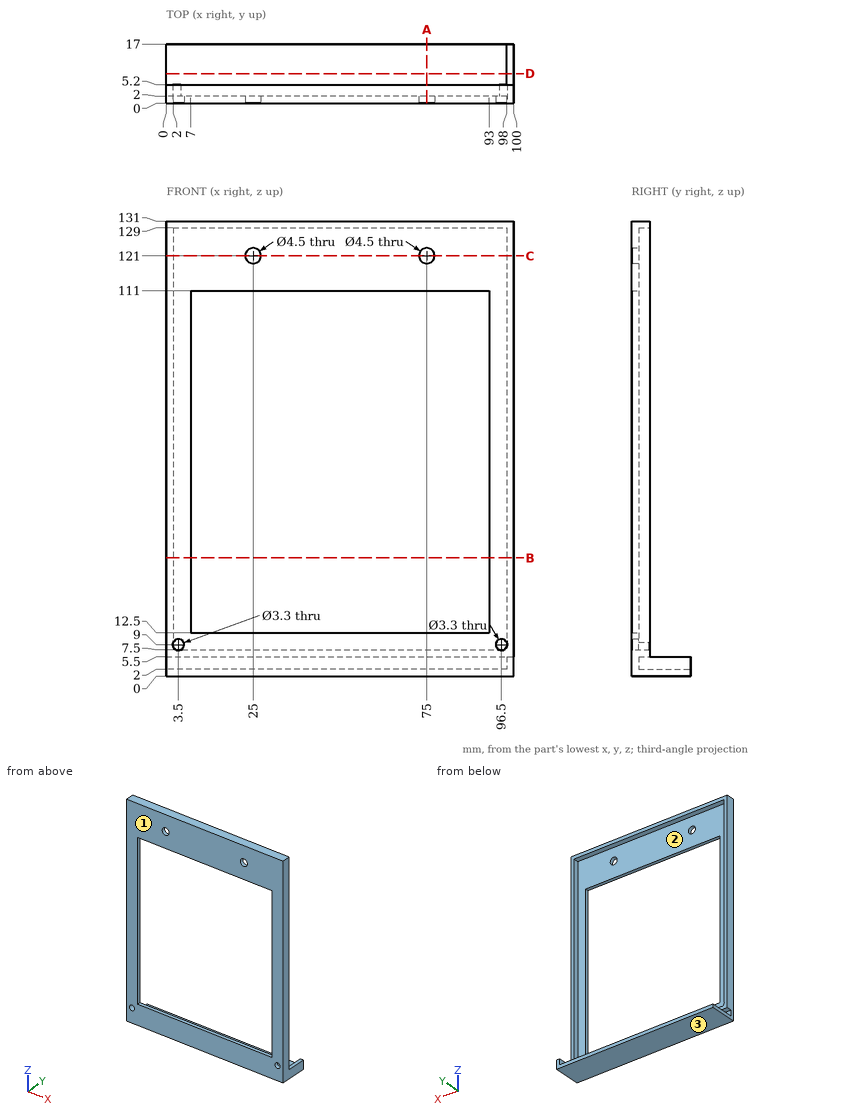
Could you check a few things on this drawing? It's one solid part, dimensions in mm from its lowest x, y, z. Give positions to 0.01 mm unless a question says otherwise; leave off trailing zeros. Write each loop counter-clockwise with the first axis right and the second up, starting at its lowest first coordinate (ties: lowest second). Pieces come first, ordered by that corner, then holes. Notation, with made-up numbers: (-12.5, 12) -> (5.5, 12) arc R19 cw to (5.5, 39) -> close; hole circle Ø7 at (-19, 57.5). An arc over 180 degrees is marked (long way). Answer as CSV lines item,"result". Start each with the question number.
(1) I'm going to push flat-ended pins straight in: pin 1 Ø4 at (x, y) = (16, 10) entering from +Z; pin 2 Ø1 at (x, z) = (34, 3.5) entering from +Y; pin 3 Ø2 at (x, y) = (99, 9) entering from +Z. Where does each tip first touch, or does it pass through?
(2) If we section it at B-B, the plane z = 34: Write out the boundary of the cut face in (x, y).
(3) If we section it at A-A, the plane x = 75: Write out the boundary of the cut face in (y, z), and give its area (3 significant figures).
(4) If we section it at C-C, the plane z = 121: Write out the boundary of the cut face in (x, y).
(5) Please list where these lines run through material, in increasing order: line 1 (X direction, y = 1.4, z = 121); line 2 (X direction, y = 1.35, z = 9); line 3 (Z direction, x = 75, y = 0.9).
(6) If we mould it in two halves opening along Z, with no side actions, what happens to the marked faces 1, 2 and 3? For each: +Z half, -Z half, draft (parallel to the pull), parting line (faces both ways), or undercut.
(7) If we section it at D-D, the plane y = 8.5: Write out the boundary of the cut face in (x, z), and give its area (3 significant figures).
Answer list:
1,pin 1,"z = 2"
1,pin 2,"y = 2"
1,pin 3,"z = 5.5"
2,outline,"(0, 0) -> (7, 0) -> (7, 2) -> (2, 2) -> (2, 5.2) -> (0, 5.2) -> close; (93, 0) -> (100, 0) -> (100, 5.2) -> (98, 5.2) -> (98, 2) -> (93, 2) -> close"
3,outline,"(0, 0) -> (17, 0) -> (17, 2) -> (2, 2) -> (2, 5.5) -> (5.2, 5.5) -> (5.2, 7.5) -> (2, 7.5) -> (2, 12.5) -> (0, 12.5) -> close; (0, 111) -> (2, 111) -> (2, 118.75) -> (0, 118.75) -> close; (0, 123.25) -> (2, 123.25) -> (2, 129) -> (5.2, 129) -> (5.2, 131) -> (0, 131) -> close"
3,area,"98.8 mm^2"
4,outline,"(0, 0) -> (22.75, 0) -> (22.75, 2) -> (2, 2) -> (2, 5.2) -> (0, 5.2) -> close; (27.25, 0) -> (72.75, 0) -> (72.75, 2) -> (27.25, 2) -> close; (77.25, 0) -> (100, 0) -> (100, 5.2) -> (98, 5.2) -> (98, 2) -> (77.25, 2) -> close"
5,line 1,"0 to 22.75, 27.25 to 72.75, 77.25 to 100"
5,line 2,"0 to 1.85, 5.15 to 94.85, 98.15 to 100"
5,line 3,"0 to 12.5, 111 to 118.75, 123.25 to 131"
6,face 1,"draft"
6,face 2,"undercut"
6,face 3,"-Z half"
7,outline,"(0, 0) -> (100, 0) -> (100, 5.5) -> (98, 5.5) -> (98, 2) -> (0, 2) -> close"
7,area,"207 mm^2"
